Read the model definition and answer for the solid it produces. Units are mm, in the model's axes. Face numbers are marked on the shaded views. A direction names the side the tool comes from. Coordinates: 2 decimals unless noted, no trailing zeros. Order: outer loops, then holes, each group sorted by start corner. A loop starts at its lowest first (then second) coordinate and runs counter-clockwise, first axis right, second up.
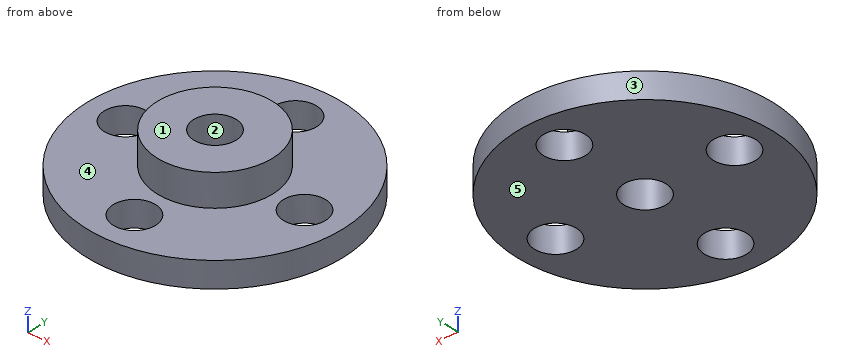
```python
from build123d import *

# Parameters (mm, degrees)
SKETCH_1_R          = 10
EXTRUDE_1_DEPTH     = 2
SKETCH_2_R          = 4.5
EXTRUDE_2_DEPTH     = 2.5
SKETCH_3_R          = 1.65
CUT_EXTRUDE_1_DEPTH = 8.5
SKETCH_4_R          = 1.65
CUT_EXTRUDE_2_DEPTH = 8.5


with BuildPart() as part:
    # 草图1 → 凸台-拉伸1 (new body)
    with BuildSketch(Plane.XY):
        Circle(SKETCH_1_R)
    extrude(amount=EXTRUDE_1_DEPTH)

    # 草图2 → 凸台-拉伸2 (add)
    with BuildSketch(Plane.XY.offset(2)):
        Circle(SKETCH_2_R)
    extrude(amount=EXTRUDE_2_DEPTH)

    # 草图3 → 切除-拉伸1 (cut)
    with BuildSketch(Plane.XY.offset(4.5)):
        Circle(SKETCH_3_R)
    extrude(amount=-CUT_EXTRUDE_1_DEPTH, mode=Mode.SUBTRACT)

    # 草图4 → 切除-拉伸2 (cut)
    with BuildSketch(Plane.XY.offset(2)):
        with Locations((0, 7)):
            Circle(SKETCH_4_R)
        with Locations((7, 0)):
            Circle(SKETCH_4_R)
        with Locations((0, -7)):
            Circle(SKETCH_4_R)
        with Locations((-7, 0)):
            Circle(SKETCH_4_R)
    extrude(amount=-CUT_EXTRUDE_2_DEPTH, mode=Mode.SUBTRACT)


solid = part.part
```
1) Which of the six approach directions +Z, -Z, +X, -X, +Y, -Y give full straight-line access (tool end or side, diameter ignored) to the marked faces 4 and 5?
A:
face 4: +Z
face 5: -Z, +X, -X, +Y, -Y
2) Straight lines are drawn through the part: line 1 (Y direction, x = 0, z = 0.45); line 2 (Z direction, x = -1.5, y = -9); line 3 (Y direction, x = -7, z = 1). For each, find the intervals that lie inside material, in ascending order.
A:
line 1: y = -10 to -8.65, -5.35 to -1.65, 1.65 to 5.35, 8.65 to 10
line 2: z = 0 to 2
line 3: y = -7.14 to -1.65, 1.65 to 7.14
3) Flat-ended cylindrical pins translate along their axes: pin 1 Ø4 at (x, y) = (2.5, 2.5) entering from -Z; pin 2 Ø1 at (x, z) = (1.5, 3.5) entering from +Y; pin 3 Ø2 at (y, z) = (-1.5, 3.5) entering from +X. Find the tip coordinate at first contact, or state that the pin passes through.
A:
pin 1: stops at z = 0
pin 2: stops at y = 4.39
pin 3: stops at x = 4.47
4) A cutting plane is placed at B-B, the plane x = -7. Determine the outline of the cut face in (y, z).
A:
outline: (-7.14, 0) - (-1.65, 0) - (-1.65, 2) - (-7.14, 2) - close; (1.65, 0) - (7.14, 0) - (7.14, 2) - (1.65, 2) - close
5) Determine the mould class of the marked faces 1, 2 and 3 for opening direction X: pulls with the +X half, pulls with the -X half, needs draft (parallel to the pull), parting line crosses it, or undercut.
A:
face 1: needs draft
face 2: undercut
face 3: parting line crosses it
6) A cutting plane is placed at D-D, the plane y = -6. Determine the outline of the cut face in (x, z).
A:
outline: (-8, 0) - (-1.31, 0) - (-1.31, 2) - (-8, 2) - close; (1.31, 0) - (8, 0) - (8, 2) - (1.31, 2) - close
7) A cutting plane is placed at C-C, the plane z = 3.9. Determine the outline of the cut face in (x, y), and give its area (3 significant figures).
A:
outline: circle Ø9 at (0, 0); hole circle Ø3.3 at (0, 0)
area: 55.1 mm2
8) A cutting plane is placed at A-A, the plane y = 0. Determine the outline of the cut face in (x, z).
A:
outline: (-10, 0) - (-8.65, 0) - (-8.65, 2) - (-10, 2) - close; (-5.35, 0) - (-1.65, 0) - (-1.65, 4.5) - (-4.5, 4.5) - (-4.5, 2) - (-5.35, 2) - close; (1.65, 0) - (5.35, 0) - (5.35, 2) - (4.5, 2) - (4.5, 4.5) - (1.65, 4.5) - close; (8.65, 0) - (10, 0) - (10, 2) - (8.65, 2) - close
